Source: three-view drawing plus pictorial views. Frame: mm from the lowest corner of the part. Round coordinates to 2 decimals unless told otherwise and drop trailing zeros. Loops run counter-clockwise (first coordinate to the right, second up) from the corner with the lowest first, then second, coordinate; pieces in that order, holes last. Notation, with made-up numbers: (7, 50) -> (26, 50) arc R20 ccw to (26, 58) -> close; hole circle Ø11 at (-3.5, 88.25). An arc over 180 degrees is marked (long way). One line per question, with ' | ' between items. Start each with the question number.
Q1. Cut plane D-D on x = 96.5. Return loops of the section in (y, z).
Q2. Cut plane A-A on x = 76.2. Return loops of the section in (y, z) (3 decimals), and give its area (3 significant figures).
Q3. Contact query for flat-ended pins moving along their axis: P1, Ø1, axis at x = 58, y = 4, coming from the +Z side; P2, Ø8, axis at x = 96, y = 28.5, coming from the +Z side; P3, Ø5, axis at y = 28, z = 72, coming from the -X side; P4, Ø4, axis at x = 76.2, z = 76.2, coming from the -Y side. Output: stop coordinate, or through.
Q4. Cut plane C-C on y = 14. Return loops of the section in (x, z) (3 decimals), and give its area (3 significant figures).
Q5. Cut plane B-B on z = 76.2. Return loops of the section in (x, y) (3 decimals).
Q6. Mould query, pull axis Z, two halves, no side actions, for the marked faces 1, 2 and 3. Classes: pulls with the +Z half, pulls with the -Z half, needs draft (parallel to the pull), parting line crosses it, or undercut.
Q7. Material intervals for L1, parallel to X at y = 36, z = 76; L2, parallel to Z at x = 76, y = 13, sorted ascending.
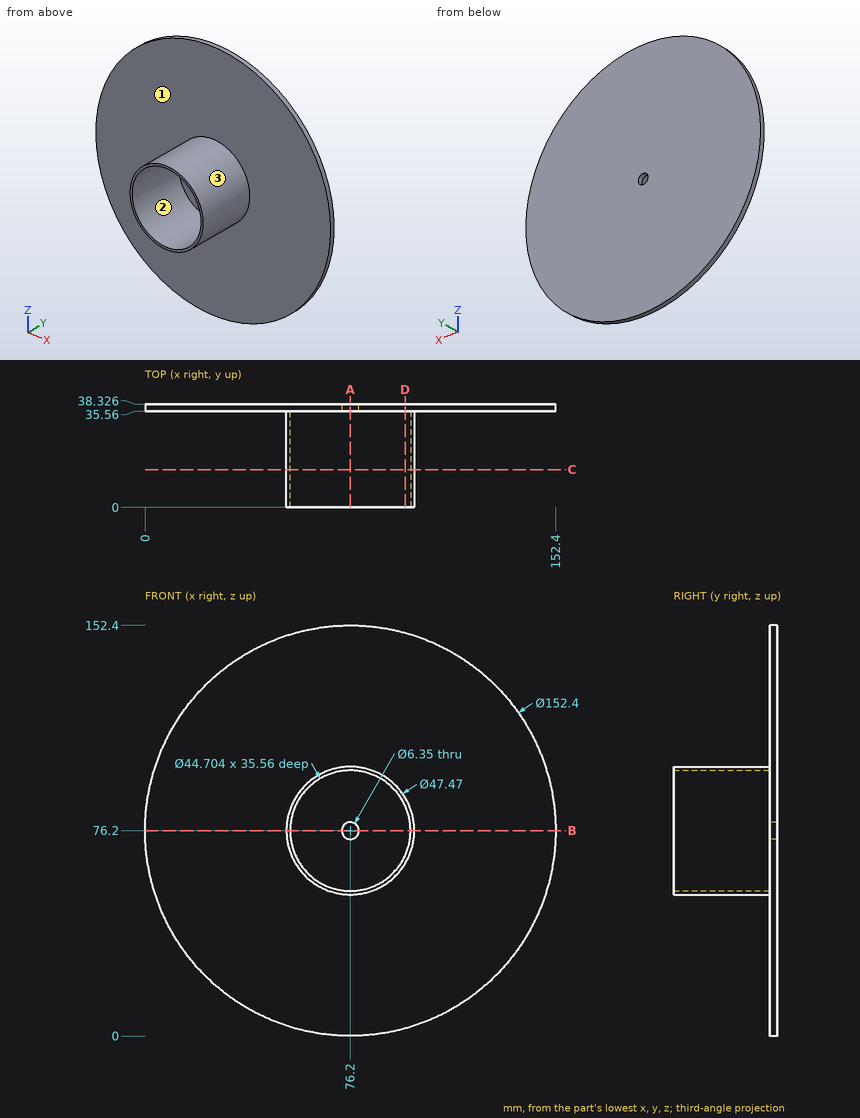
Results:
1) outline: (0, 63.9) -> (35.56, 63.9) -> (35.56, 2.75) -> (38.33, 2.75) -> (38.33, 149.65) -> (35.56, 149.65) -> (35.56, 88.5) -> (0, 88.5) -> (0, 85.56) -> (35.56, 85.56) -> (35.56, 66.84) -> (0, 66.84) -> close
2) outline: (0, 52.465) -> (35.56, 52.465) -> (35.56, 0) -> (38.326, 0) -> (38.326, 73.025) -> (35.56, 73.025) -> (35.56, 53.848) -> (0, 53.848) -> close; (0, 98.552) -> (35.56, 98.552) -> (35.56, 79.375) -> (38.326, 79.375) -> (38.326, 152.4) -> (35.56, 152.4) -> (35.56, 99.935) -> (0, 99.935) -> close | area: 502 mm^2
3) P1: z = 92.01 | P2: z = 93.91 | P3: x = 52.53 | P4: through
4) outline: circle Ø47.47 at (76.2, 76.2); hole circle Ø44.704 at (76.2, 76.2) | area: 200 mm^2
5) outline: (0, 35.56) -> (52.465, 35.56) -> (52.465, 0) -> (53.848, 0) -> (53.848, 35.56) -> (73.025, 35.56) -> (73.025, 38.326) -> (0, 38.326) -> close; (79.375, 35.56) -> (98.552, 35.56) -> (98.552, 0) -> (99.935, 0) -> (99.935, 35.56) -> (152.4, 35.56) -> (152.4, 38.326) -> (79.375, 38.326) -> close
6) face 1: needs draft | face 2: undercut | face 3: parting line crosses it
7) L1: 0 to 73.03, 79.37 to 152.4 | L2: 52.47 to 53.85, 98.55 to 99.93
